Autodesk Inventor part; units mm, degrees
ref_plane "YZ Plane" through (0, 0, 0) normal (1, 0, 0) x (0, 1, 0)
ref_plane "XZ Plane" through (0, 0, 0) normal (0, 1, 0) x (-1, 0, 0)
ref_plane "XY Plane" through (0, 0, 0) normal (0, 0, 1) x (1, 0, 0)
sketch "草圖1" plane through (0, 0, 0) normal (1, 0, 0) x (0, 1, 0)
  line L0 (0, 0) -> (0, 32)
  line L1 (0, 32) -> (4, 32)
  line L2 (4, 32) -> (4, 4)
  line L3 (4, 4) -> (21, 4)
  line L4 (21, 4) -> (21, 0)
  line L5 (21, 0) -> (0, 0)
  dimension "d0" = 32
  dimension "d1" = 21
  dimension "d2" = 4
  dimension "d3" = 4
extrude "擠出1" add sketch "草圖1" along normal blind 12.5
sketch "草圖2" plane through (0, 4, 32) normal (0, 1, 0) x (1, 0, 0)
  circle A0 centre (6.25, 11.88) radius 2.5
  line L0 (0, 0) -> (12.5, 0)
  point P0 (0, 32)
  dimension "d6" = 5
  dimension "d7" = 11.88
extrude "擠出2" cut sketch "草圖2" against normal blind 12.5
sketch "草圖3" plane through (0, 4, 4) normal (0, 0, 1) x (1, 0, 0)
  circle A0 centre (6.25, 7) radius 4
  line L0 (0, 0) -> (0, 17)
  line L1 (0, -4) -> (12.5, -4)
  dimension "d10" = 8
  dimension "d11" = 6.25
  dimension "d12" = 11
extrude "擠出3" cut sketch "草圖3" against normal blind 12.5
properties part number "L形件"
Part model, mm, in its own coordinate system. A direction names the side the tool comes from. Give positions to 0.01 mm unless a question says otherwise; leave off trailing zeros. Order: outer loops, then holes, each group sorted by start corner. A loop starts at its lowest first (then second) coordinate and runs counter-clockwise, first axis right, second up. Notation, with made-up numbers: (30, 40) - (58, 40) arc R19 cw to (58, 59) - close; hole circle Ø8 at (45, 79). An arc over 180 degrees is marked (long way). Use one line per item in the form item = value.
Item 1: Probe probe 1 along X at (y, z) = (1, 20.12); probe 2 along Y at (x, z) = (6.25, 2.2); probe 3 along Z at (x, y) = (6.25, 1.95). List the from-to ranges inside material, lowest first. Write a range as from..to.
Solution:
probe_1 = 0..3.75, 8.75..12.5
probe_2 = 0..7, 15..21
probe_3 = 0..17.62, 22.62..32
Item 2: Pin check, flat tips, straight feed: pin 1 Ø5 at (x, z) = (5.5, 9.5) entering from +Y; pin 2 Ø1 at (x, z) = (7, 23) entering from -Y; pin 3 Ø4 at (x, y) = (5, 9) entering from +Z. Stop position of each tip, or through.
Solution:
pin_1 = 4
pin_2 = 0
pin_3 = 4
Item 3: Which spindle directions (+Z, -Z, +X, -X, +Y, -Y) get a long thin tool onto all of the face, cutting with end or side? Do faces 4 (the face through (8.9, 14.3, 4)), 5 (the face through (12.5, 3, 14)). Say none if no direction does.
Solution:
face_4 = +Z, +X, -X, +Y
face_5 = +Z, -Z, +X, +Y, -Y
Item 4: Slice it at D-D on y = 2.5. Give the cut face in (x, z).
Solution:
outline = (0, 0) - (12.5, 0) - (12.5, 32) - (0, 32) - close; hole circle Ø5 at (6.25, 20.12)
Item 5: Slice it at C-C on y = 11. Give the cut face in (x, z), and give its area (3 significant figures).
Solution:
outline = (0, 0) - (2.25, 0) - (2.25, 4) - (0, 4) - close; (10.25, 0) - (12.5, 0) - (12.5, 4) - (10.25, 4) - close
area = 18.0 mm2
Item 6: Slice it at B-B on z = 20.12. Give the cut face in (x, y), and give its area (3 significant figures).
Solution:
outline = (0, 0) - (3.75, 0) - (3.75, 4) - (0, 4) - close; (8.75, 0) - (12.5, 0) - (12.5, 4) - (8.75, 4) - close
area = 30.0 mm2
Item 7: Slice it at A-A on x = 6.25. Give the cut face in (y, z), and give its area (3 significant figures).
Solution:
outline = (0, 0) - (7, 0) - (7, 4) - (4, 4) - (4, 17.62) - (0, 17.62) - close; (0, 22.62) - (4, 22.62) - (4, 32) - (0, 32) - close; (15, 0) - (21, 0) - (21, 4) - (15, 4) - close
area = 144 mm2
Item 8: Two-plate mould, pull along X, no slides. Class faces 1 (the face through (5.729, 14.966, 2.028)), 2 (the face through (3, 4, 18)), 3 (the face through (0, 3, 14)): released by +X, released by -X, zero draft, split by the parting line, or undercut.
Solution:
face_1 = undercut
face_2 = zero draft
face_3 = released by -X
